For this review, take the finished solid that the model builds, in its own axes (mm). Face numbers are marked on the shaded views. A direction names the side the tool comes from. Coordinates: 2 decimals unless noted, no trailing zeros. Write each loop counter-clockwise with the first axis right and the second up, starting at its lowest first coordinate (ties: lowest second). Pieces come first, ordered by that corner, then holes.
1) We need section D-D on y = 58.5. Write out the cut boundary in (x, z), then the cut area to 3 significant figures.
2) We need section C-C on x = 56.5. Write out the cut boundary in (y, z), then the cut area to 3 significant figures.
3) For the marked faces 1 and 2, list the 3-axis set-ups (+Z, -Z, +X, -X, +Y, -Y) from which the entire face can be reached by the end or side of a thin tool; tool diameter is ignored.
4) We need section B-B on z = 37.5. Write out the cut boundary in (x, y), then the cut area to 3 significant figures.
5) To check wall thickness, follow line 1 along X through (y, z) = (24, 25); line 2 along Z through (x, y) = (75, 19); line 3 along X through (y, z) = (47.5, 6). State the ranges of each line that lie inside material, in increasing order.
6) Insertion check: P1, Ø15, axis at x = 83, z = 21, coming from the +Y side. The pin has a flat end and moves straight along its axis. Give the tip position at first contact, or say it passes through.
7) We need section A-A on y = 22. Write out the cut boundary in (x, z), then the cut area to 3 significant figures.
from build123d import *

# Parameters (mm, degrees)
F0_W     = 100
F0_H     = 80
F1_DEPTH = 50
F2_W     = 50
F2_H     = 50
F3_DEPTH = 50
F4_SIZE  = 20
F7_DEPTH = 80.001


with BuildPart() as f1:
    # F0 (on Top) → F1 (new body)
    with BuildSketch(Plane.XY):
        with Locations((50, 40)):
            Rectangle(F0_W, F0_H)
    extrude(amount=F1_DEPTH)

    # F2 (on face) → F3 (cut, through all)
    with BuildSketch(Plane.XY.offset(50)):
        with Locations((75, 55)):
            Rectangle(F2_W, F2_H)
    extrude(amount=-F3_DEPTH, mode=Mode.SUBTRACT)

    # F4
    f4_edges = [f1.edges().sort_by_distance(p)[0] for p in [
        (0, 80, 25),
    ]]
    chamfer(f4_edges, length=F4_SIZE)

    # F6 (on face) → F7 (cut, through all)
    with BuildSketch(Plane.XZ):
        with BuildLine():
            ThreePointArc((82.5, 25), (69.696699, 30.303301), (75, 17.5))
            ThreePointArc((75, 17.5), (80.303301, 19.696699), (82.5, 25))
        make_face()
    extrude(amount=-F7_DEPTH, mode=Mode.SUBTRACT)


solid = f1.part
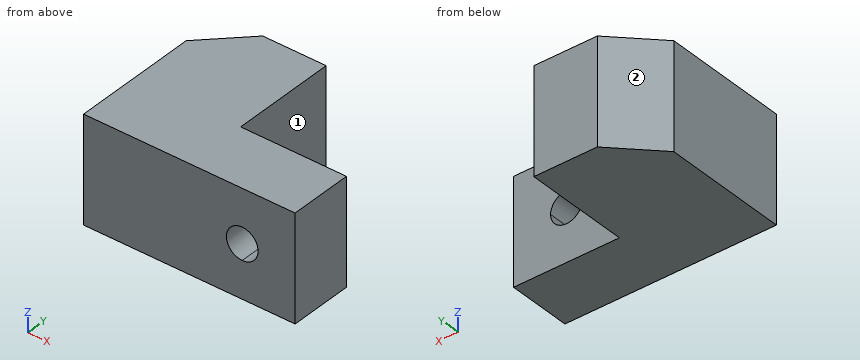
Result:
1. outline: (0, 0) - (50, 0) - (50, 50) - (0, 50) - close
1. area: 2,500 mm2
2. outline: (0, 0) - (30, 0) - (30, 50) - (0, 50) - close
2. area: 1,500 mm2
3. face 1: +Z, -Z, +X, +Y
3. face 2: +Z, -Z, -X, +Y
4. outline: (0, 0) - (100, 0) - (100, 30) - (50, 30) - (50, 80) - (20, 80) - (0, 60) - close
4. area: 5,300 mm2
5. line 1: x = 0 to 67.5, 82.5 to 100
5. line 2: z = 0 to 17.5, 32.5 to 50
5. line 3: x = 0 to 50
6. P1: stops at y = 30
7. outline: (0, 0) - (100, 0) - (100, 50) - (0, 50) - close; hole circle Ø15 at (75, 25)
7. area: 4,820 mm2
